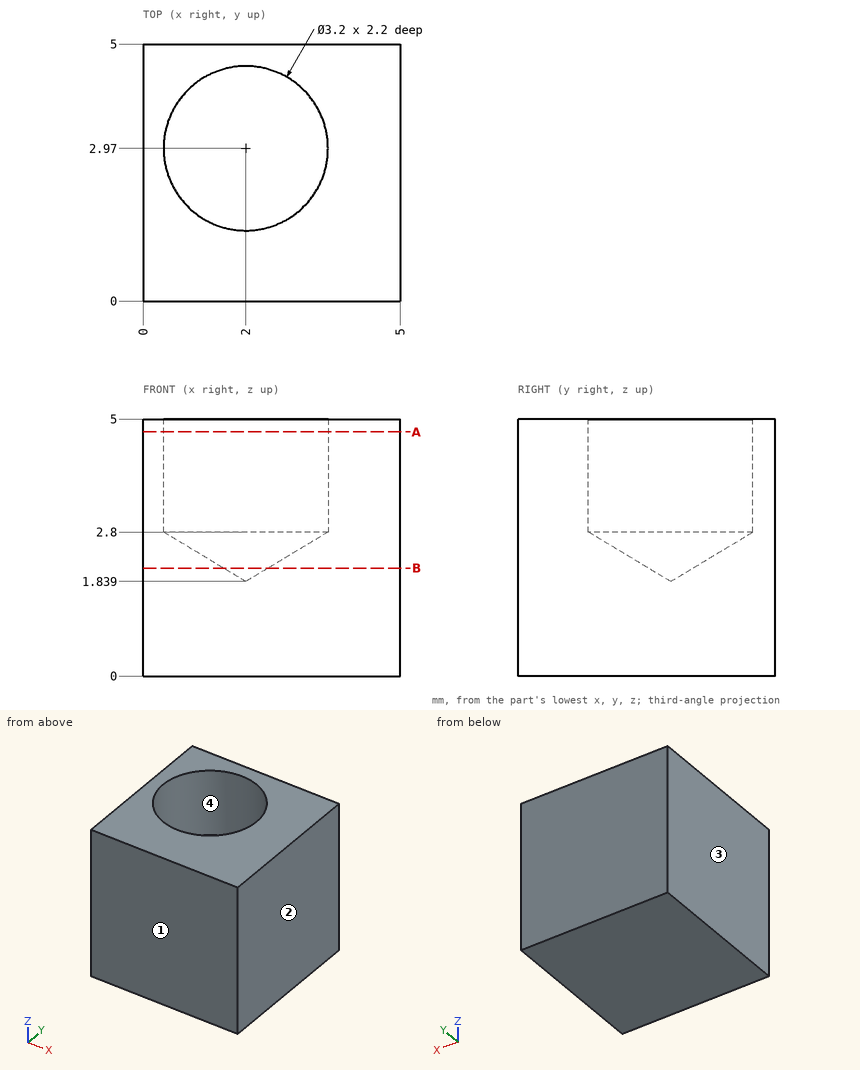
Here's the drawing with two shaded views (mm, measured from the low corner). I have some questions. Round coordinates to 2 decimals unless told otherwise and drop trailing zeros. Loops run counter-clockwise (first coordinate to the right, second up) from the corner with the lowest first, then second, coordinate; pieces in that order, holes last.
1. Thinking about a two-plate mould opening in X: for the marked faces 1, 2, 3 and 4, which applies, released by +X, released by -X, zero draft, split by the parting line, or undercut?
Answers:
face 1: zero draft
face 2: released by +X
face 3: released by -X
face 4: undercut
2. Suppose I cut it at A-A, the plane z = 4.75. Please give me the cut outline in (x, y).
Answers:
outline: (0, 0) - (5, 0) - (5, 5) - (0, 5) - close; hole circle Ø3.2 at (2, 2.97)
3. Suppose I cut it at B-B, the plane z = 2.1. Please give me the cut outline in (x, y) (1 decimal).
Answers:
outline: (0, 0) - (5, 0) - (5, 5) - (0, 5) - close; hole circle Ø0.9 at (2, 3)
4. Will this pin go through, and if not, where does the flat tip stop? pin 1 (3 mm diameter, centred on x = 2, y = 2.97, fed in from +Z).
Answers:
pin 1: stops at z = 2.74
5. If I drill on probe 1 along Y at (x, z) = (2, 3.65); probe 2 along Y at (x, z) = (3.4, 4.65) (1 decimal); probe 3 along X at (y, z) = (2.65, 4.4), over which ranges is the centre line in solid material (lowest first)?
Answers:
probe 1: y = 0 to 1.37, 4.57 to 5
probe 2: y = 0 to 2.2, 3.7 to 5
probe 3: x = 0 to 0.43, 3.57 to 5
